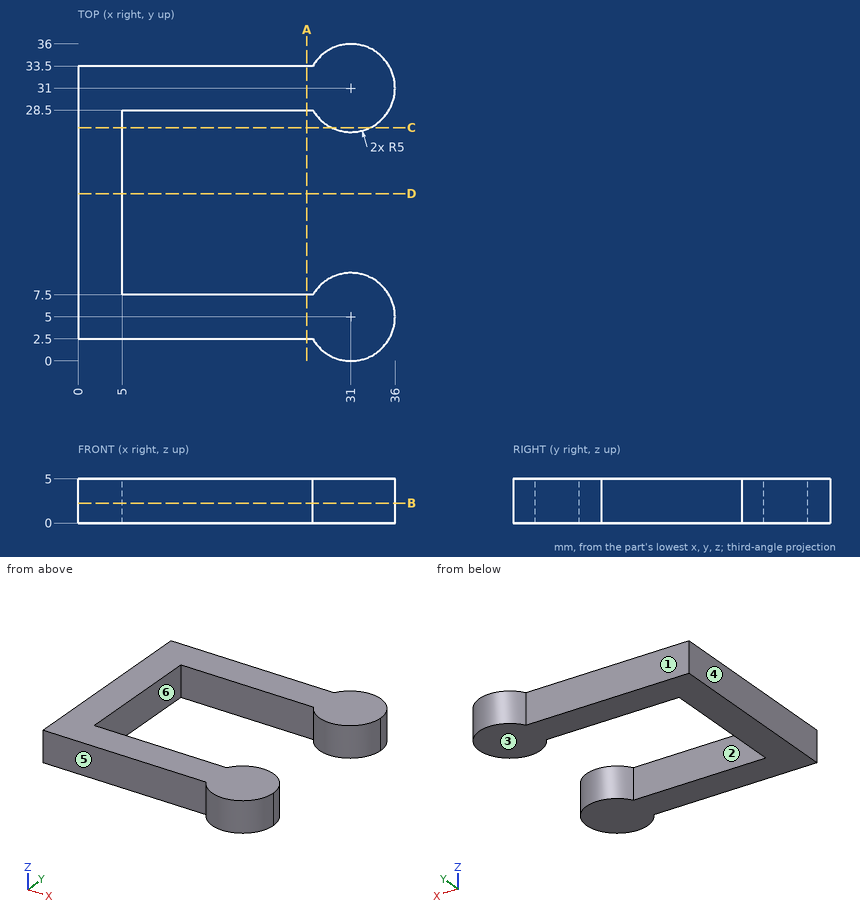
Geometry check sheet. Reference: drawing and pictorial views, mm from the part's lowest x, y, z. A direction names the side the tool comes from. Give positions to 0.01 mm unless a question says otherwise; leave off trailing zeros. Order: outer loops, then holes, each group sorted by start corner. A loop starts at its lowest first (then second) coordinate and runs counter-clockwise, first axis right, second up. Notation, with made-up numbers: (-24.5, 58.5) - (5.5, 58.5) arc R31 ccw to (5.5, 87.5) - close; hole circle Ø1 at (-12, 70.5). An arc over 180 degrees is marked (long way). Answer as CSV lines item,"result".
1. Go/stop test with a flat-tipped pin: P1, Ø1.5, axis at y = 14.5, z = 2, coming from the +X side. Record where the tip stops, or that it passes through.
Result sheet:
P1,"x = 5"
2. Tool access check on the marked faces 1, 2 and 3. Record the directions out of +Z, -Z, +X, -X, +Y, -Y that give a thin tool (end or side, any length) a straight path to the whole face; none if there is none.
Result sheet:
face 1,"+Z, -Z, -X, +Y"
face 2,"+Z, -Z"
face 3,"-Z, +X, -X, +Y, -Y"
3. Section check B-B (z = 2.25). Record the boundary of the cut face in (x, y).
Result sheet:
outline,"(0, 2.5) - (26.67, 2.5) arc R5 ccw (long way) to (26.67, 7.5) - (5, 7.5) - (5, 28.5) - (26.67, 28.5) arc R5 ccw (long way) to (26.67, 33.5) - (0, 33.5) - close"
4. Scan lines: probe 1 along Y at (x, z) = (5.5, 0.9); probe 2 along Y at (x, z) = (2, 1); probe 3 along X at (y, z) = (19, 3.7). Record each from-to range of solid material in increasing order. Write a range as from..to.
Result sheet:
probe 1,"2.5..7.5, 28.5..33.5"
probe 2,"2.5..33.5"
probe 3,"0..5"
5. Section check A-A (x = 26). Record the boundary of the cut face in (y, z).
Result sheet:
outline,"(2.5, 0) - (7.5, 0) - (7.5, 5) - (2.5, 5) - close; (28.5, 0) - (33.5, 0) - (33.5, 5) - (28.5, 5) - close"
6. Section check C-C (y = 26.5). Record the boundary of the cut face in (x, z), then the cut area to 3 significant figures.
Result sheet:
outline,"(0, 0) - (5, 0) - (5, 5) - (0, 5) - close; (28.82, 0) - (33.18, 0) - (33.18, 5) - (28.82, 5) - close"
area,"46.8 mm²"
7. Mould release check, pull along X, two halves, no side actions. Record for the marked faces 4, 5 and 6: released by +X, released by -X, zero draft, split by the parting line, or undercut.
Result sheet:
face 4,"released by -X"
face 5,"zero draft"
face 6,"undercut"
8. Section check D-D (y = 19). Record the boundary of the cut face in (x, z), then the cut area to 3 significant figures.
Result sheet:
outline,"(0, 0) - (5, 0) - (5, 5) - (0, 5) - close"
area,"25.0 mm²"
